Model file for the job. Use its own axes, mm. A direction names the side the tool comes from. Give positions to 0.01 mm unless a question says otherwise; leave off trailing zeros. Write each loop counter-clockwise with the first axis right and the second up, starting at its lowest first coordinate (ties: lowest second). Pieces come first, ordered by that corner, then holes. Notation, with made-up numbers: (33, -9.75) - (86, -9.75) arc R25 cw to (86, 17.25) - close; hole circle Ø10 at (85.5, 0). An arc over 180 degrees is marked (long way). One line per item, written item: value. Start each with the question number.
(1) Cut at A-A, the plane z = 69. List the corners of the cut face in (x, y).
(2) Drop flat-ended pins along their axis: P1, Ø2, axis at x = -1, y = 1, coming from the +Z side; P2, Ø4, axis at y = 1, z = 142.5, coming from the +X side; P3, Ø1, axis at x = 1, y = -1.5, coming from the -Z side (3 decimals). Give the stop position or say it passes through.
(3) Mould opens along Y. For faces 1 (the face through (-2, 3, 0)), 2 (the face through (-0.86, -3.874, 1.174)), 3 (the face through (-0.69, 3.1, 1.57)) say: pulls with the +Y half, pulls with the -Y half, needs draft (parallel to the pull), parting line crosses it, or undercut.
(4) Probe L1, parallel to X at y = 0, z = 1.7 (3 decimals); L2, parallel to X at y = -1, z = 32. List the from-to ranges inside material, lowest first.
(5) 3-axis set-ups, long thin cutter, end or side, ignore diameter. For faces 4 (the face through (0, 0, 3.175)), 5 (the face through (-3.45, -1.96, 5.12)), 6 (the face through (0, 1, 34.925)): which of +Z, -Z, +X, -X, +Y, -Y reach the whole face in a straight line?
from build123d import *

# Parameters (mm, degrees)
F0_R      = 3.96875
F1_DEPTH  = 2.38125
F3_DEPTH  = 5.55625
F4_R      = 3.96875
F5_DEPTH  = 1.5875
F6_R      = 3.175
F7_DEPTH  = 3.175
F8_R      = 1.5875
F9_DEPTH  = 25.4
F12_R     = 0.79375
F13_DEPTH = 144.4625


# Not quite as in the source:
# - a length typed as a fraction of an inch, garbled in the dataset ("3 / 203.2 mm" for 3/8 in), is restored


with BuildPart() as f1:
    # F0 (on Top) → F1 (new body)
    with BuildSketch(Plane.XY):
        Circle(F0_R)
    extrude(amount=F1_DEPTH)

    # F2 (on face) → F3 (join)
    with BuildSketch(Plane.XY.offset(2.38125)):
        Polygon((2.2913588808, 3.96875), (-2.2913588808, 3.96875), (-4.5827177617, 0), (-2.2913588808, -3.96875), (2.2913588808, -3.96875), (4.5827177617, 0), align=None)
    extrude(amount=F3_DEPTH)

    # F4 (on face) → F5 (join)
    with BuildSketch(Plane.XY.offset(7.9375)):
        Circle(F4_R)
    extrude(amount=F5_DEPTH)

    # F6 (on face) → F7 (cut)
    with BuildSketch(Plane(origin=(0, 0, 0), x_dir=(1, 0, 0), z_dir=(0, 0, -1))):
        Circle(F6_R)
    extrude(amount=-F7_DEPTH, mode=Mode.SUBTRACT)

    # F8 (on face) → F9 (join)
    with BuildSketch(Plane.XY.offset(9.525)):
        Circle(F8_R)
    extrude(amount=F9_DEPTH)

    # F10 (on Front) → F11 (revolve)
    with BuildSketch(Plane.XZ):
        Polygon((1.5875, 34.925), (0, 34.925), (0, 9.525), (3.9187353296, 9.525), align=None)
    revolve(axis=Axis((0, 0, 9.525), (0, 0, 1)))

    # F12 (on face) → F13 (join)
    with BuildSketch(Plane.XY.offset(34.925)):
        Circle(F12_R)
    extrude(amount=F13_DEPTH)


solid = f1.part
Answers follow:
1. outline: circle Ø1.59 at (0, 0)
2. P1: stops at z = 179.39
2. P2: stops at x = 0.79
2. P3: stops at z = 3.175
3. face 1: needs draft
3. face 2: parting line crosses it
3. face 3: undercut
4. L1: x = -3.969 to -3.175, 3.175 to 3.969
4. L2: x = -1.56 to 1.56
5. face 4: -Z
5. face 5: +Z, -Z, -X, -Y
5. face 6: +Z
